Design review of the part built by this model. Coordinates are the model's own, in mm. Coordinates: 2 decimals unless noted, no trailing zeros. Order: outer loops, then holes, each group sorted by start corner. A loop starts at its lowest first (then second) coordinate and runs counter-clockwise, first axis right, second up.
from build123d import *

# Parameters (mm, degrees)
F0_R     = 4
F0_W     = 3
F0_H     = 75
F1_DEPTH = 3


with BuildPart() as f1:
    # F0 (on Front) → F1 (new body)
    with BuildSketch(Plane.XZ):
        with BuildLine():
            Line((-181.5, -70), (181.5, -70))
            ThreePointArc((181.5, -70), (183.62132, -69.12132), (184.5, -67))
            Line((184.5, -67), (184.5, 67))
            ThreePointArc((184.5, 67), (183.62132, 69.12132), (181.5, 70))
            Line((181.5, 70), (-181.5, 70))
            ThreePointArc((-181.5, 70), (-183.62132, 69.12132), (-184.5, 67))
            Line((-184.5, 67), (-184.5, -67))
            ThreePointArc((-184.5, -67), (-183.62132, -69.12132), (-181.5, -70))
        make_face()
        with Locations((-132.5, -45)):
            Circle(F0_R, mode=Mode.SUBTRACT)
        with Locations((132.5, -45)):
            Circle(F0_R, mode=Mode.SUBTRACT)
        with Locations((-153, 0)):
            Rectangle(F0_W, F0_H, mode=Mode.SUBTRACT)
        with Locations((-132.5, 45)):
            Circle(F0_R, mode=Mode.SUBTRACT)
        with BuildLine():
            ThreePointArc((125, -22), (124.12132, -24.12132), (122, -25))
            Line((122, -25), (-122, -25))
            ThreePointArc((-122, -25), (-124.12132, -24.12132), (-125, -22))
            Line((-125, -22), (-125, 22))
            ThreePointArc((-125, 22), (-124.12132, 24.12132), (-122, 25))
            Line((-122, 25), (122, 25))
            ThreePointArc((122, 25), (124.12132, 24.12132), (125, 22))
            Line((125, 22), (125, -22))
        make_face(mode=Mode.SUBTRACT)
        with Locations((153, 0)):
            Rectangle(F0_W, F0_H, mode=Mode.SUBTRACT)
        with Locations((132.5, 45)):
            Circle(F0_R, mode=Mode.SUBTRACT)
    extrude(amount=F1_DEPTH)


solid = f1.part
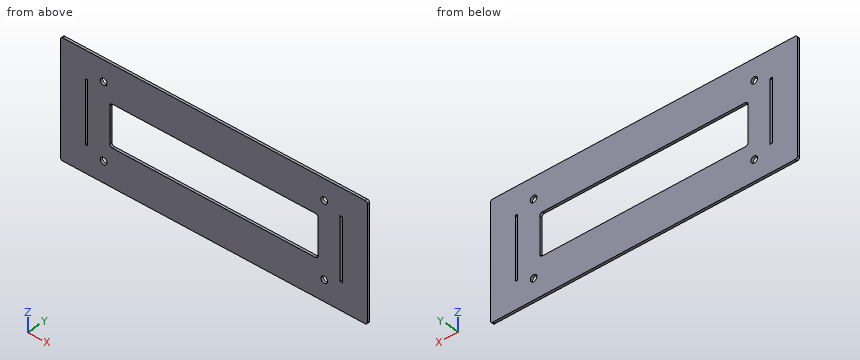
1. Add section C-C (z = 1). Give the boundary of the cut face in (x, y).
2. Insertion check: pin 1 (5 mm diameter, centred on x = -132.5, z = 45, fed in from +Y); pin 2 (9 mm diameter, centred on x = 132.5, z = 45, fed in from +Y). Each pin has a flat end and moves straight along its axis. Give the tip position at first contact, or say it passes through.
3. Add section A-A (z = 45). Give the boundary of the cut face in (x, y), and give its area (3 significant figures).
4. Add section B-B (x = 74). Give the boundary of the cut face in (y, z), and give its area (3 significant figures).
5. To check wall thickness, follow line 1 (X direction, y = -0.3, z = 22); line 2 (Z direction, x = 132.5, y = -0.9); line 3 (Z direction, x = 73, y = -0.3). State the ranges of each line that lie inside material, in increasing order.
6. Add section D-D (x = 132.5). Give the boundary of the cut face in (y, z).
Solution:
1. outline: (-184.5, -3) - (-154.5, -3) - (-154.5, 0) - (-184.5, 0) - close; (-151.5, -3) - (-125, -3) - (-125, 0) - (-151.5, 0) - close; (125, -3) - (151.5, -3) - (151.5, 0) - (125, 0) - close; (154.5, -3) - (184.5, -3) - (184.5, 0) - (154.5, 0) - close
2. pin 1: passes through
2. pin 2: stops at y = 0
3. outline: (-184.5, -3) - (-136.5, -3) - (-136.5, 0) - (-184.5, 0) - close; (-128.5, -3) - (128.5, -3) - (128.5, 0) - (-128.5, 0) - close; (136.5, -3) - (184.5, -3) - (184.5, 0) - (136.5, 0) - close
3. area: 1,060 mm2
4. outline: (-3, -70) - (0, -70) - (0, -25) - (-3, -25) - close; (-3, 25) - (0, 25) - (0, 70) - (-3, 70) - close
4. area: 270 mm2
5. line 1: x = -184.5 to -154.5, -151.5 to -125, 125 to 151.5, 154.5 to 184.5
5. line 2: z = -70 to -49, -41 to 41, 49 to 70
5. line 3: z = -70 to -25, 25 to 70
6. outline: (-3, -70) - (0, -70) - (0, -49) - (-3, -49) - close; (-3, -41) - (0, -41) - (0, 41) - (-3, 41) - close; (-3, 49) - (0, 49) - (0, 70) - (-3, 70) - close
